Design review of the part built by this model. Coordinates are the model's own, in mm. A direction names the side the tool comes from. Give positions to 0.01 mm unless a question says otherwise; leave off trailing zeros. Order: outer loops, then holes, each group sorted by start corner. A loop starts at its lowest first (then second) coordinate and runs counter-clockwise, first axis right, second up. Notation, with made-up numbers: M -21.75,10 L 33.25,10 A29 cw 33.25,38 Z; hole C 19,-5 d1. An arc over 180 degrees is marked long. Answer as a JSON object with one key per item and string values.
from build123d import *

# Parameters (mm, degrees)
PAD_DEPTH       = 75
SKETCH001_R     = 3
POCKET_DEPTH    = 110.001
SKETCH002_R     = 2.1
POCKET001_DEPTH = 6
SKETCH003_W     = 26.5
SKETCH003_H     = 52
POCKET002_DEPTH = 2
FILLET_R        = 10
FILLET001_R     = 3
FILLET002_R     = 2
FILLET003_R     = 2


with BuildPart() as part:
    # Sketch → Pad (new body, symmetric)
    with BuildSketch(Plane.XY):
        Polygon((0, 40), (-100, 40), (-100, 0), (-110, 0), (-110, 50), (0, 50), align=None)
        Polygon((0, 40), (0, 50), align=None)
    extrude(amount=PAD_DEPTH, both=True)

    # Sketch001 (on Face3 of Pad) → Pocket (cut, through all)
    with BuildSketch(Plane(origin=(-110, 0, 0), x_dir=(0, -1, 0), z_dir=(-1, 0, 0))):
        with Locations((-20, -50)):
            Circle(SKETCH001_R)
        with Locations((-20, 50)):
            Circle(SKETCH001_R)
    extrude(amount=-POCKET_DEPTH, mode=Mode.SUBTRACT)

    # Sketch002 → Pocket001 (cut)
    with BuildSketch(Plane.XZ.offset(-40)):
        with Locations((-24.5, 29)):
            Circle(SKETCH002_R)
        with Locations((-24.5, -29)):
            Circle(SKETCH002_R)
    extrude(amount=-POCKET001_DEPTH, mode=Mode.SUBTRACT)

    # Sketch003 (on Face2 of Pocket001) → Pocket002 (cut)
    with BuildSketch(Plane.XZ.offset(-40)):
        with Locations((-13.25, 0)):
            Rectangle(SKETCH003_W, SKETCH003_H)
    extrude(amount=-POCKET002_DEPTH, mode=Mode.SUBTRACT)

    # Fillet
    fillet_edges = [part.edges().sort_by_distance(p)[0] for p in [
        (-105, 0, -75),
        (-105, 0, 75),
        (-110, 50, 0),
    ]]
    fillet(fillet_edges, radius=FILLET_R)

    # Fillet001
    fillet001_edges = [part.edges().sort_by_distance(p)[0] for p in [
        (-100, 40, 0),
    ]]
    fillet(fillet001_edges, radius=FILLET001_R)

    # Fillet002
    fillet002_edges = [part.edges().sort_by_distance(p)[0] for p in [
        (-110, 25, -75),
        (-100, 23.5, -75),
    ]]
    fillet(fillet002_edges, radius=FILLET002_R)

    # Fillet003
    fillet003_edges = [part.edges().sort_by_distance(p)[0] for p in [
        (-26.5, 41, 26),
        (-26.5, 41, -26),
    ]]
    fillet(fillet003_edges, radius=FILLET003_R)

    # Mirrored: part across YZ


with BuildPart() as part_1:
    add(part.part)
    add(part.part.mirror(Plane.YZ))


solid = part_1.part
(1) We need section C-C (x = -74). Write out the cut boundary in (y, z).
Checked values:
{"outline": "M 40,-73 A2 ccw 42,-75 L 48,-75 A2 ccw 50,-73 L 50,73 A2 ccw 48,75 L 42,75 A2 ccw 40,73 Z"}
(2) We need section D-D (z = -14.5). Write out the cut boundary in (x, y), plus the area to 3 significant figures.
Checked values:
{"outline": "M -110,2 A2 ccw -108,0 L -102,0 A2 ccw -100,2 L -100,37 A3 cw -97,40 L -26.5,40 L -26.5,42 L 26.5,42 L 26.5,40 L 97,40 A3 cw 100,37 L 100,2 A2 ccw 102,0 L 108,0 A2 ccw 110,2 L 110,40 A10 ccw 100,50 L -100,50 A10 ccw -110,40 Z", "area": "2,850 mm^2"}
(3) To check wall thickness, follow L1, parallel to Z at x = -24.5, y = 43.05; L2, parallel to Z at x = 24.5, y = 41.9; L3, parallel to X at y = 12.5, z = 30. State the ranges of each line that lie inside material, in increasing order. Write a range as from..to.
Checked values:
{"L1": "z = -75..-31.1, -26.9..26.9, 31.1..75", "L2": "z = -75..-31.1, -26.9..-26, 26..26.9, 31.1..75", "L3": "x = -110..-100, 100..110"}
(4) We need section A-A (y = 20). Count the separate pieces of the cut face and the enclosed holes in it, plus the area to 3 significant figures.
Checked values:
{"separate pieces": "6", "enclosed holes": "0", "area": "2,750 mm^2"}
(5) Insertion check: pin 1 (1.5 mm diameter, centred on x = -19.5, z = 4.5, fed in from -Y); pin 2 (3.5 mm diameter, centred on x = -24.5, z = 28.5, fed in from -Y); pin 3 (5.5 mm diameter, centred on y = 20, z = -50, fed in from +X); pin 4 (6 mm diameter, centred on y = 40.5, z = 2.5, fed in from +X). Each pin has a flat end and moves straight along its axis. Give the tip position at first contact, or say it passes through.
Checked values:
{"pin 1": "stops at y = 42", "pin 2": "stops at y = 40", "pin 3": "passes through", "pin 4": "stops at x = 110"}
(6) Tool access review of faces 4 (the flat face through (-100, 20, 1)), 5 (the cylindrical face through (-105.04, 3.01, 72.15)), 6 (the cylindrical face through (23.531, 42.958, 27.137)): name each direction out of +Z, -Z, +X, -X, +Y, -Y from which nothing blocks a thin tool from reaching the whole face with its end or side.
Checked values:
{"face 4": "+Z, -Z, -Y", "face 5": "+Z, +X, -X, -Y", "face 6": "-Y"}
(7) Draft analysis for pull direction Y (two halves, no side actions). For faces 1 (the cylindrical face through (105, 20, 53)), 2 (the flat face through (25, 46, -29)), 3 (the flat face through (-1, 43, -75)), state which applies: +Y half, -Y half, draft (parallel to the pull), parting line (faces both ways), or undercut.
Checked values:
{"face 1": "undercut", "face 2": "-Y half", "face 3": "draft"}
(8) We need section B-B (z = 50). Write out the cut boundary in (x, y).
Checked values:
{"outline": "M -110,2 A2 ccw -108,0 L -102,0 A2 ccw -100,2 L -100,17 L -110,17 Z; M -110,23 L -100,23 L -100,37 A3 cw -97,40 L 97,40 A3 cw 100,37 L 100,23 L 110,23 L 110,40 A10 ccw 100,50 L -100,50 A10 ccw -110,40 Z; M 100,2 A2 ccw 102,0 L 108,0 A2 ccw 110,2 L 110,17 L 100,17 Z"}
